from build123d import *

# Parameters (mm, degrees)
SKETCH1_W           = 220
SKETCH1_H           = 220
BOSS_EXTRUDE1_DEPTH = 4.5
CUT_EXTRUDE1_REACH  = 6.5
SKETCH2_R           = 13
CUT_EXTRUDE2_REACH  = 6.5
SKETCH3_R           = 2.75
CUT_EXTRUDE3_REACH  = 6.5
SKETCH4_R           = 2.5


with BuildPart() as part:
    # Sketch1 → Boss-Extrude1 (new body)
    with BuildSketch(Plane(origin=(0, 0, 0), x_dir=(1, 0, 0), z_dir=(0, 1, 0))):
        Rectangle(SKETCH1_W, SKETCH1_H)
    extrude(amount=BOSS_EXTRUDE1_DEPTH)

    # Sketch2 → Cut-Extrude1 (cut, up to next)
    with BuildSketch(Plane(origin=(0, 4.5, 0), x_dir=(1, 0, 0), z_dir=(0, 1, 0)), mode=Mode.PRIVATE) as cut_extrude1_sk1:
        with Locations((-20, -50)):
            Circle(SKETCH2_R)
    cut_extrude1_tool1 = extrude(cut_extrude1_sk1.sketch, amount=-CUT_EXTRUDE1_REACH, mode=Mode.PRIVATE) & part.part
    add(cut_extrude1_tool1.solids().sort_by_distance((-20, 4.5, 50))[0], mode=Mode.SUBTRACT)

    # Sketch3 → Cut-Extrude2 (cut, up to next)
    with BuildSketch(Plane(origin=(0, 4.5, 0), x_dir=(1, 0, 0), z_dir=(0, 1, 0)), mode=Mode.PRIVATE) as cut_extrude2_sk1:
        with Locations((-95, -93)):
            Circle(SKETCH3_R)
    cut_extrude2_tool1 = extrude(cut_extrude2_sk1.sketch, amount=-CUT_EXTRUDE2_REACH, mode=Mode.PRIVATE) & part.part
    add(cut_extrude2_tool1.solids().sort_by_distance((-95, 4.5, 93))[0], mode=Mode.SUBTRACT)
    # Sketch3 → Cut-Extrude2 (cut, up to next)
    with BuildSketch(Plane(origin=(0, 4.5, 0), x_dir=(1, 0, 0), z_dir=(0, 1, 0)), mode=Mode.PRIVATE) as cut_extrude2_sk2:
        with Locations((70, -93)):
            Circle(SKETCH3_R)
    cut_extrude2_tool2 = extrude(cut_extrude2_sk2.sketch, amount=-CUT_EXTRUDE2_REACH, mode=Mode.PRIVATE) & part.part
    add(cut_extrude2_tool2.solids().sort_by_distance((70, 4.5, 93))[0], mode=Mode.SUBTRACT)

    # Sketch4 → Cut-Extrude3 (cut, up to next)
    with BuildSketch(Plane(origin=(0, 0, 0), x_dir=(-1, 0, 0), z_dir=(0, -1, 0)), mode=Mode.PRIVATE) as cut_extrude3_sk1:
        with Locations((-60, 96)):
            Circle(SKETCH4_R)
    cut_extrude3_tool1 = extrude(cut_extrude3_sk1.sketch, amount=-CUT_EXTRUDE3_REACH, mode=Mode.PRIVATE) & part.part
    add(cut_extrude3_tool1.solids().sort_by_distance((60, 0, -96))[0], mode=Mode.SUBTRACT)
    # Sketch4 → Cut-Extrude3 (cut, up to next)
    with BuildSketch(Plane(origin=(0, 0, 0), x_dir=(-1, 0, 0), z_dir=(0, -1, 0)), mode=Mode.PRIVATE) as cut_extrude3_sk2:
        with Locations((60, 97.5)):
            Circle(SKETCH4_R)
    cut_extrude3_tool2 = extrude(cut_extrude3_sk2.sketch, amount=-CUT_EXTRUDE3_REACH, mode=Mode.PRIVATE) & part.part
    add(cut_extrude3_tool2.solids().sort_by_distance((-60, 0, -97.5))[0], mode=Mode.SUBTRACT)


solid = part.part
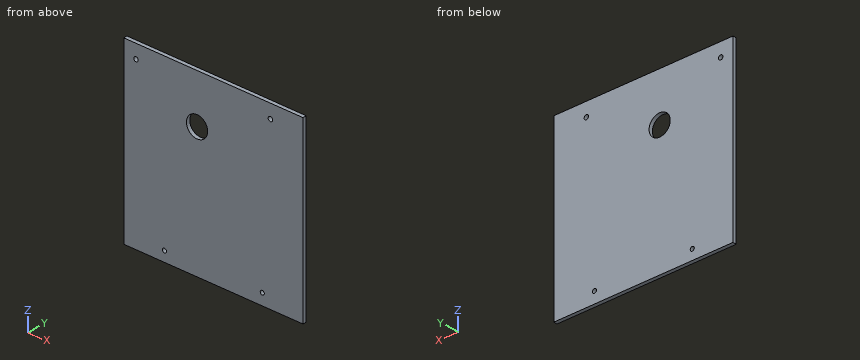
Design review of the part built by this model. Coordinates are the model's own, in mm. Give positions to 0.01 mm unless a question says otherwise; leave off trailing zeros. Order: outer loops, then holes, each group sorted by start corner. A loop starts at its lowest first (then second) coordinate and runs counter-clockwise, first axis right, second up.
1. Add section A-A, the plane z = 50. State the section outline as (x, y) points.
Solution:
outline: (-110, 0) - (-33, 0) - (-33, 4.5) - (-110, 4.5) - close; (-7, 0) - (110, 0) - (110, 4.5) - (-7, 4.5) - close
2. Add section B-B, the plane x = 70. State the section outline as (y, z) points, then the cut area to 3 significant figures.
Solution:
outline: (0, -110) - (4.5, -110) - (4.5, 90.25) - (0, 90.25) - close; (0, 95.75) - (4.5, 95.75) - (4.5, 110) - (0, 110) - close
area: 965 mm2
3. For pin 1 Ø3 at (x, z) = (60, -96) entering from +Y, flat-tipped, find the tip position at first contact; note if it passes through.
Solution:
pin 1: passes through
4. Add section C-C, the plane z = 93. State the section outline as (x, y) points.
Solution:
outline: (-110, 0) - (-97.75, 0) - (-97.75, 4.5) - (-110, 4.5) - close; (-92.25, 0) - (67.25, 0) - (67.25, 4.5) - (-92.25, 4.5) - close; (72.75, 0) - (110, 0) - (110, 4.5) - (72.75, 4.5) - close
5. To check wall thickness, follow L1, parallel to X at y = 2.3, z = 93; L2, parallel to X at y = 2.2, z = -96; L3, parallel to Z at x = -60, y = 2.6. State the ranges of each line that lie inside material, in increasing order.
Solution:
L1: x = -110 to -97.75, -92.25 to 67.25, 72.75 to 110
L2: x = -110 to -62, -58 to 57.5, 62.5 to 110
L3: z = -110 to -100, -95 to 110
